from build123d import *

# Parameters (mm, degrees)
BOSS_EXTRUDE1_DEPTH   = 28
BOSS_EXTRUDE1_2_DEPTH = 28
SKETCH1_3_R           = 36
BOSS_EXTRUDE2_DEPTH   = 55
CUT_EXTRUDE1_START    = 55
SKETCH1_4_R           = 25
CUT_EXTRUDE1_DEPTH    = 12
CUT_EXTRUDE2_START    = 31
SKETCH1_5_W           = 26
SKETCH1_5_H           = 85.646984924
CUT_EXTRUDE2_DEPTH    = 64.21915941
SKETCH2_W             = 18
SKETCH2_H             = 32
CUT_EXTRUDE3_DEPTH    = 20


with BuildPart() as part:
    # Sketch1 → Boss-Extrude1 (new body)
    with BuildSketch(Plane(origin=(0, 0, 0), x_dir=(1, 0, 0), z_dir=(0, 1, 0))):
        with BuildLine():
            ThreePointArc((36, 0), (32.485281374, -15.514718626), (22.627416998, -28))
            Line((22.627416998, -28), (67.5, -28))
            Line((67.5, -28), (67.5, 28))
            Line((67.5, 28), (22.627416998, 28))
            ThreePointArc((22.627416998, 28), (32.485281374, 15.514718626), (36, 0))
        make_face()
    extrude(amount=BOSS_EXTRUDE1_DEPTH)



with BuildPart() as body_2:
    # Sketch1 → Boss-Extrude1 2 (new body)
    with BuildSketch(Plane(origin=(0, 0, 0), x_dir=(1, 0, 0), z_dir=(0, 1, 0))):
        with BuildLine():
            Line((-67.5, 28), (-67.5, -28))
            Line((-67.5, -28), (-22.627416998, -28))
            ThreePointArc((-22.627416998, -28), (-36, 0), (-22.627416998, 28))
            Line((-22.627416998, 28), (-67.5, 28))
        make_face()
    extrude(amount=BOSS_EXTRUDE1_2_DEPTH)


with BuildPart() as part_1:
    add(part.part)

    add(body_2.part)  # Boss-Extrude2 merges body 2
    # Sketch1_3 → Boss-Extrude2 (add)
    with BuildSketch(Plane(origin=(0, 0, 0), x_dir=(1, 0, 0), z_dir=(0, 1, 0))):
        with Locations(Location((0, 0, 0), (0, 0, 128.942441269))):
            Circle(SKETCH1_3_R)
    extrude(amount=BOSS_EXTRUDE2_DEPTH)

    # Sketch1_4 → Cut-Extrude1 (cut)
    with BuildSketch(Plane(origin=(0, 0, 0), x_dir=(1, 0, 0), z_dir=(0, 1, 0)).offset(CUT_EXTRUDE1_START)):
        with Locations(Location((0, 0, 0), (0, 0, 270))):
            Circle(SKETCH1_4_R)
    extrude(amount=-CUT_EXTRUDE1_DEPTH, mode=Mode.SUBTRACT)

    # Sketch1_5 → Cut-Extrude2 (cut, through all)
    with BuildSketch(Plane(origin=(0, 0, 0), x_dir=(1, 0, 0), z_dir=(0, 1, 0)).offset(CUT_EXTRUDE2_START)):
        Rectangle(SKETCH1_5_W, SKETCH1_5_H)
    extrude(amount=CUT_EXTRUDE2_DEPTH, mode=Mode.SUBTRACT)

    # Sketch2 → Cut-Extrude3 (cut)
    with BuildSketch(Plane(origin=(0, 28, 0), x_dir=(1, 0, 0), z_dir=(0, 1, 0))):
        with Locations((-58.5, 0)):
            Rectangle(SKETCH2_W, SKETCH2_H)
        with Locations((58.5, 0)):
            Rectangle(SKETCH2_W, SKETCH2_H)
    extrude(amount=-CUT_EXTRUDE3_DEPTH, mode=Mode.SUBTRACT)


solid = part_1.part
Work out the finished part from the listing and answer in its coordinate system (mm). A direction names the side the tool comes from. Give positions to 0.01 mm unless a question says otherwise; leave off trailing zeros. Loops run counter-clockwise (first coordinate to the right, second up) from the corner with the lowest first, then second, coordinate; pieces in that order, holes last. Notation, with made-up numbers: (20, 85) -> (38, 85) arc R17 cw to (38, 103) -> close; hole circle Ø4 at (-33.75, 58). An arc over 180 degrees is marked (long way). Use a Markdown table: item, result. Add a question column.
1. Find the intervals of material crossed by probe 1 along X at (y, z) = (37, -13); probe 2 along Z at (x, y) = (-48, 18.5); probe 3 along Y at (x, z) = (-16.5, -14), in increasing order.
2. Section C-C on z = 0 is taken. Determine the outline of the cut face in (x, y), and give its area (3 significant figures).
3. Section A-A on y = 45 is taken. Determine the outline of the cut face in (x, z), and give its area (3 significant figures).
4. Section D-D on y = 23 is taken. Determine the outline of the cut face in (x, z).
5. Section B-B on x = 56.5 is taken. Determine the outline of the cut face in (y, z), and give its area (3 significant figures).
6. Flat-ended cylindrical pins translate along their axes: pin 1 Ø1 at (x, z) = (53, 15) entering from +Y; pin 2 Ø12 at (y, z) = (48, -7.5) entering from -X; pin 3 Ø9 at (x, y) = (62.5, 15.5) entering from +Z. Find the tip coordinate at first contact, or state that the pin passes through.
7. Determine the mould class of faces 1 (the cylindrical face through (34.994, 33.226, 8.451)), 2 (the flat face through (-18, 43, 0)), 3 (the flat face through (0, 31, -1)) for opening direction Z: released by +Z, released by -Z, zero draft, split by the parting line, or undercut.
8. For faces 4 (the cylindrical face through (25, 49, 0)), 5 (the flat face through (-45, 14, -28)), 6 (the flat face through (58, 8, 0)), 7 (the flat face through (-59, 8, 0)), 8 (the flat face through (13, 40, 0)), determine the directions among +Z, -Z, +X, -X, +Y, -Y from which every point of the face is accessible in a straight line to the end or side of a thin tool.
Results below:
| question | item | result |
|---|---|---|
| 1 | probe 1 | x = -33.57 to -13, 13 to 33.57 |
| 1 | probe 2 | z = -28 to 28 |
| 1 | probe 3 | y = 0 to 43 |
| 2 | outline | (-67.5, 0) -> (67.5, 0) -> (67.5, 8) -> (49.5, 8) -> (49.5, 28) -> (36, 28) -> (36, 55) -> (25, 55) -> (25, 43) -> (13, 43) -> (13, 31) -> (-13, 31) -> (-13, 43) -> (-25, 43) -> (-25, 55) -> (-36, 55) -> (-36, 28) -> (-49.5, 28) -> (-49.5, 8) -> (-67.5, 8) -> close |
| 2 | area | 4,090 mm^2 |
| 3 | outline | (-13, -33.57) -> (-13, -21.35) arc R25 cw to (-13, 21.35) -> (-13, 33.57) arc R36 ccw to start; (13, -33.57) arc R36 ccw to (13, 33.57) -> (13, 21.35) arc R25 cw to (13, -21.35) -> close |
| 3 | area | 1,520 mm^2 |
| 4 | outline | (-67.5, -28) -> (-22.63, -28) arc R36 ccw to (22.63, -28) -> (67.5, -28) -> (67.5, -16) -> (49.5, -16) -> (49.5, 16) -> (67.5, 16) -> (67.5, 28) -> (22.63, 28) arc R36 ccw to (-22.63, 28) -> (-67.5, 28) -> (-67.5, 16) -> (-49.5, 16) -> (-49.5, -16) -> (-67.5, -16) -> close |
| 5 | outline | (0, -28) -> (28, -28) -> (28, -16) -> (8, -16) -> (8, 16) -> (28, 16) -> (28, 28) -> (0, 28) -> close |
| 5 | area | 928 mm^2 |
| 6 | pin 1 | stops at y = 8 |
| 6 | pin 2 | stops at x = -35.97 |
| 6 | pin 3 | stops at z = 28 |
| 7 | face 1 | split by the parting line |
| 7 | face 2 | undercut |
| 7 | face 3 | zero draft |
| 8 | face 4 | +Y |
| 8 | face 5 | -Z, -X, +Y, -Y |
| 8 | face 6 | +X, +Y |
| 8 | face 7 | -X, +Y |
| 8 | face 8 | +Z, -Z, +Y |
